Could you check a few things on this model? Use its own coordinates, in mm. Coordinates: 2 decimals unless noted, no trailing zeros. Loops run counter-clockwise (first coordinate to the right, second up) from the corner with the lowest first, then second, coordinate; pieces in that order, holes last.
from build123d import *

# Parameters (mm, degrees)
SKETCH2_W           = 193
SKETCH2_H           = 93
BOSS_EXTRUDE1_DEPTH = 3
SKETCH3_R           = 1.5
SKETCH3_W           = 40
SKETCH3_H           = 3
SKETCH3_W_2         = 3
SKETCH3_H_2         = 20
CUT_EXTRUDE1_DEPTH  = 3


with BuildPart() as part:
    # Sketch2 → Boss-Extrude1 (new body)
    with BuildSketch(Plane.XY):
        Rectangle(SKETCH2_W, SKETCH2_H)
    extrude(amount=BOSS_EXTRUDE1_DEPTH)

    # Sketch3 → Cut-Extrude1 (cut)
    with BuildSketch(Plane(origin=(0, 0, 0), x_dir=(-1, 0, 0), z_dir=(0, 0, -1))):
        with Locations((-20, 33.5)):
            Circle(SKETCH3_R)
        with Locations((10.759, 8.837)):
            Circle(SKETCH3_R)
        with Locations((-76.5, 45)):
            Rectangle(SKETCH3_W, SKETCH3_H)
        with Locations((76.5, -45)):
            Rectangle(SKETCH3_W, SKETCH3_H)
        with Locations((76.5, 45)):
            Rectangle(SKETCH3_W, SKETCH3_H)
        with Locations((0, 45)):
            Rectangle(SKETCH3_W, SKETCH3_H)
        with Locations((0, -45)):
            Rectangle(SKETCH3_W, SKETCH3_H)
        with Locations((-76.5, -45)):
            Rectangle(SKETCH3_W, SKETCH3_H)
        with Locations((95, 0)):
            Rectangle(SKETCH3_W_2, SKETCH3_H_2)
        with Locations((-95, 0)):
            Rectangle(SKETCH3_W_2, SKETCH3_H_2)
    extrude(amount=-CUT_EXTRUDE1_DEPTH, mode=Mode.SUBTRACT)


solid = part.part
(1) Imagine slicing it at A-A, the plane z = 1.2. State how many separate pieces and enclosed holes the cut face has, and give its area (3 significant figures).
Answers:
separate pieces: 1
enclosed holes: 2
area: 17,100 mm2
(2) For pin 1 (0.9 mm diameter, centred on y = 44.5, z = 1.5, fed in from -X); pin 2 (0.9 mm diameter, centred on y = -44.5, z = 1, fed in from +X); pin 3 (0.9 mm diameter, centred on x = -9.5, z = 2, fed in from -Y); pin 4 (1.8 mm diameter, centred on x = 20, y = 33.5, fed in from -Z), each with a flat end and sliding along its axis, tell me the tip position at first contact or that it passes through.
Answers:
pin 1: stops at x = -56.5
pin 2: stops at x = 56.5
pin 3: stops at y = -43.5
pin 4: passes through
(3) I need wall thicknesses on probe 1 along Y at (x, z) = (-6, 2.3); probe 2 along X at (y, z) = (4, 0.7). Which ranges of each line are inside material? Lowest first, please.
Answers:
probe 1: y = -43.5 to 43.5
probe 2: x = -93.5 to 93.5
(4) Imagine slicing it at C-C, the plane y = -2.5. Write out the boundary of the cut face in (x, z), and give its area (3 significant figures).
Answers:
outline: (-93.5, 0) - (93.5, 0) - (93.5, 3) - (-93.5, 3) - close
area: 561 mm2
(5) Imagine slicing it at B-B, the plane x = 78. Write out the boundary of the cut face in (y, z).
Answers:
outline: (-43.5, 0) - (43.5, 0) - (43.5, 3) - (-43.5, 3) - close
